The model under review builds one solid part; all positions refer to its coordinate system, in mm. A direction names the side the tool comes from. Round coordinates to 2 decimals unless told otherwise and drop trailing zeros. Loops run counter-clockwise (first coordinate to the right, second up) from the corner with the lowest first, then second, coordinate; pieces in that order, holes last. Notation, with made-up numbers: M 53,19 L 77,19 A12 ccw 77,37 Z; hole C 61.25,46.5 d11. An arc over 180 degrees is marked long. Answer as a JSON object with one key per item and string values. Group by question number.
Item 1: Consider section D-D (x = 12.5). Give the boundary of the cut face in (y, z), and give its area (3 significant figures).
Item 2: To check wall thickness, follow line 1 (X direction, y = 23, z = 3.5) (3 decimals); line 2 (X direction, y = 13.5, z = -3); line 3 (Y direction, x = -28.5, z = 0). State the ranges of each line that lie inside material, in increasing order.
Item 3: Insertion check: P1, Ø12, axis at x = -20, y = 19, coming from the +Z side; P2, Ø6, axis at y = 19.4, z = 0, coming from the -X side; P3, Ø1.5, axis at x = 18, y = 16.5, coming from the +Z side. Each pin has a flat end and moves straight along its axis. Give the tip position at first contact, or say it passes through.
Item 4: Consider section C-C (y = 17.5). Give the boundary of the cut face in (x, z), and give its area (3 significant figures).
Item 5: Consider section B-B (y = 11.5). Give the boundary of the cut face in (x, z).
Item 6: Consider section A-A (z = 0). Give the boundary of the cut face in (x, y) (3 decimals), and give its area (3 significant figures).
Item 7: Tool access review of faces 4 (the face through (20.5, 14, 0)), 5 (the face through (31, 25, 0)), 6 (the face through (29.4, 15, 0)), 7 (the face through (38.5, 13, 0)), 8 (the face through (26.355, 24, 0)): name each direction out of +Z, -Z, +X, -X, +Y, -Y from which nothing blocks a thin tool from reaching the whole face with its end or side.
Item 8: The part is to be moulded in two halves that separate along Y. For faces 1 (the face through (30.972, 24.357, 0.651)), 2 (the face through (35, 18.385, 0)), 3 (the face through (32.5, 24.6, 0)), say which applies: +Y half, -Y half, draft (parallel to the pull), parting line (faces both ways), or undercut.
```python
from build123d import *

# Parameters (mm, degrees)
SKETCH1_W           = 65
SKETCH1_H           = 12
BOSS_EXTRUDE1_DEPTH = 25
SKETCH2_R           = 5
CUT_EXTRUDE1_DEPTH  = 70.899928469
SKETCH3_W           = 41
SKETCH3_H           = 12
CUT_EXTRUDE2_DEPTH  = 15
BOSS_EXTRUDE2_START = -3.1
SKETCH5_R           = 5
SKETCH5_R_2         = 3.725
BOSS_EXTRUDE2_DEPTH = 8.9
SKETCH4_W           = 3.0500066
SKETCH4_H           = 7.5
CUT_EXTRUDE3_DEPTH  = 4.84
BOSS_EXTRUDE5_START = 6
BOSS_EXTRUDE5_DEPTH = 6
SKETCH13_W          = 1
SKETCH13_H          = 5
BOSS_EXTRUDE6_DEPTH = 11.106510599
SKETCH14_W          = 5
SKETCH14_H          = 5
BOSS_EXTRUDE7_DEPTH = 4.491999938


with BuildPart() as part:
    # Sketch1 → Boss-Extrude1 (new body)
    with BuildSketch(Plane(origin=(0, 0, 0), x_dir=(1, 0, 0), z_dir=(0, 1, 0))):
        Rectangle(SKETCH1_W, SKETCH1_H)
    extrude(amount=BOSS_EXTRUDE1_DEPTH)

    # Sketch2 → Cut-Extrude1 (cut, through all)
    with BuildSketch(Plane(origin=(32.5, 0, 0), x_dir=(0, 0, -1), z_dir=(1, 0, 0))):
        with Locations((0, 19.399202688)):
            Circle(SKETCH2_R)
    extrude(amount=-CUT_EXTRUDE1_DEPTH, mode=Mode.SUBTRACT)

    # Sketch3 → Cut-Extrude2 (cut)
    with BuildSketch(Plane(origin=(0, 25, 0), x_dir=(1, 0, 0), z_dir=(0, 1, 0))):
        Rectangle(SKETCH3_W, SKETCH3_H)
    extrude(amount=-CUT_EXTRUDE2_DEPTH, mode=Mode.SUBTRACT)

    # Sketch5 → Boss-Extrude2 (add)
    with BuildSketch(Plane(origin=(32.5, 0, 0), x_dir=(0, 0, -1), z_dir=(1, 0, 0)).offset(BOSS_EXTRUDE2_START)):
        with Locations((0, 19.399202688)):
            Circle(SKETCH5_R)
        with Locations((0, 19.399202688)):
            Circle(SKETCH5_R_2, mode=Mode.SUBTRACT)
    extrude(amount=-BOSS_EXTRUDE2_DEPTH)

    # Sketch4 → Cut-Extrude3 (cut)
    with BuildSketch(Plane(origin=(0, 25, 0), x_dir=(1, 0, 0), z_dir=(0, 1, 0))):
        with Locations((27.88, 0)):
            Rectangle(SKETCH4_W, SKETCH4_H)
    extrude(amount=-CUT_EXTRUDE3_DEPTH, mode=Mode.SUBTRACT)

    # Sketch12 → Boss-Extrude5 (add)
    with BuildSketch(Plane(origin=(32.5, 0, 0), x_dir=(0, 0, -1), z_dir=(1, 0, 0)).offset(BOSS_EXTRUDE5_START)):
        with BuildLine():
            Line((-2.5, 25), (-6, 25))
            Line((-6, 25), (-6, 0))
            Line((-6, 0), (6, 0))
            Line((6, 0), (6, 25))
            Line((6, 25), (2.5, 25))
            Line((2.5, 25), (2.5, 23.729329707))
            ThreePointArc((2.5, 23.729329707), (4.330127019, 21.899202688), (5, 19.399202688))
            ThreePointArc((5, 19.399202688), (4.330127019, 16.899202688), (2.5, 15.069075669))
            Line((2.5, 15.069075669), (2.5, 13.893489401))
            Line((2.5, 13.893489401), (-2.5, 13.893489401))
            Line((-2.5, 13.893489401), (-2.5, 15.069075669))
            ThreePointArc((-2.5, 15.069075669), (-5, 19.399202688), (-2.5, 23.729329707))
            Line((-2.5, 23.729329707), (-2.5, 25))
        make_face()
        with BuildLine():
            Line((-2.5, 15.069075669), (-2.5, 23.729329707))
            ThreePointArc((-2.5, 23.729329707), (-5, 19.399202688), (-2.5, 15.069075669))
        make_face()
        with BuildLine():
            ThreePointArc((5, 19.399202688), (4.330127019, 21.899202688), (2.5, 23.729329707))
            Line((2.5, 23.729329707), (2.5, 15.069075669))
            ThreePointArc((2.5, 15.069075669), (4.330127019, 16.899202688), (5, 19.399202688))
        make_face()
    extrude(amount=-BOSS_EXTRUDE5_DEPTH)

    # Sketch13 → Boss-Extrude6 (add)
    with BuildSketch(Plane(origin=(0, 25, 0), x_dir=(1, 0, 0), z_dir=(0, 1, 0))):
        with Locations((38, 0)):
            Rectangle(SKETCH13_W, SKETCH13_H)
    extrude(amount=-BOSS_EXTRUDE6_DEPTH)

    # Sketch14 → Boss-Extrude7 (add)
    with BuildSketch(Plane(origin=(0, 13.893489401, 0), x_dir=(1, 0, 0), z_dir=(0, 1, 0))):
        with Locations((35, 0)):
            Rectangle(SKETCH14_W, SKETCH14_H)
    extrude(amount=BOSS_EXTRUDE7_DEPTH)


solid = part.part
```
Geometry results:
{
 "1": {"outline": "M 0,-6 L 10,-6 L 10,6 L 0,6 Z", "area": "120 mm^2"},
 "2": {"line 1": "x = -32.5 to -20.5, 20.5 to 26.355, 29.405 to 38.5", "line 2": "x = -32.5 to -20.5, 20.5 to 38.5", "line 3": "y = 0 to 14.4, 24.4 to 25"},
 "3": {"P1": "stops at z = 6", "P2": "stops at x = 32.5", "P3": "passes through"},
 "4": {"outline": "M -32.5,-6 L -20.5,-6 L -20.5,-4.63 L -32.5,-4.63 Z; M -32.5,4.63 L -20.5,4.63 L -20.5,6 L -32.5,6 Z; M 20.5,-6 L 38.5,-6 L 38.5,6 L 20.5,6 L 20.5,3.2 L 29.4,3.2 L 29.4,4.63 L 32.5,4.63 L 32.5,-4.63 L 29.4,-4.63 L 29.4,-3.2 L 20.5,-3.2 Z", "area": "163 mm^2"},
 "5": {"outline": "M -32.5,-6 L -20.5,-6 L -20.5,6 L -32.5,6 Z; M 20.5,-6 L 38.5,-6 L 38.5,6 L 20.5,6 Z"},
 "6": {"outline": "M -32.5,0 L 38.5,0 L 38.5,25 L 37.5,25 L 37.5,18.385 L 32.5,18.385 L 32.5,14.399 L 29.4,14.399 L 29.4,15.674 L 20.5,15.674 L 20.5,10 L -20.5,10 L -20.5,14.399 L -32.5,14.399 Z; M -32.5,24.399 L -20.5,24.399 L -20.5,25 L -32.5,25 Z; M 20.5,23.124 L 26.355,23.124 L 26.355,25 L 20.5,25 Z; M 29.405,24.399 L 32.5,24.399 L 32.5,25 L 29.405,25 Z", "area": "904 mm^2"},
 "7": {"face 4": "+Z, -Z, +Y", "face 5": "+Z, -Z, +X, -X, +Y", "face 6": "none", "face 7": "+Z, -Z, +X, +Y, -Y", "face 8": "+Y"},
 "8": {"face 1": "undercut", "face 2": "+Y half", "face 3": "draft"}
}
